```python
from build123d import *

# Parameters (mm, degrees)
RESSALTO_EXTRUS_O1_DEPTH = 3
ESBO_O2_R                = 2.5
RESSALTO_EXTRUS_O2_DEPTH = 18
ESBO_O3_R                = 0.85
CORTE_EXTRUS_O1_DEPTH    = 39.774991941
ESBO_O4_R                = 0.7
CORTE_EXTRUS_O2_DEPTH    = 38.235735524


with BuildPart() as part:
    # Esboço1 → Ressalto-extrusão1 (new body)
    with BuildSketch(Plane(origin=(0, 0, 0), x_dir=(0, 0, -1), z_dir=(1, 0, 0))):
        with BuildLine():
            Line((-30, 2.5), (30, 2.5))
            ThreePointArc((30, 2.5), (32.5, 0), (30, -2.5))
            Line((30, -2.5), (-30, -2.5))
            ThreePointArc((-30, -2.5), (-32.5, 0), (-30, 2.5))
        make_face()
    extrude(amount=RESSALTO_EXTRUS_O1_DEPTH)

    # Esboço2 → Ressalto-extrusão2 (add)
    with BuildSketch(Plane(origin=(3, 0, 0), x_dir=(0, 0, -1), z_dir=(1, 0, 0))):
        with Locations(Location((30, 0, 0), (0, 0, 90))):
            Circle(ESBO_O2_R)
    extrude(amount=RESSALTO_EXTRUS_O2_DEPTH)

    # Esboço3 → Corte-extrusão1 (cut, through all)
    with BuildSketch(Plane(origin=(21, 0, 0), x_dir=(0, 0, -1), z_dir=(1, 0, 0))):
        with Locations((30, 0)):
            Circle(ESBO_O3_R)
    extrude(amount=-CORTE_EXTRUS_O1_DEPTH, mode=Mode.SUBTRACT)

    # Esboço4 → Corte-extrusão2 (cut, through all)
    with BuildSketch(Plane(origin=(3, 0, 0), x_dir=(0, 0, -1), z_dir=(1, 0, 0))):
        with Locations((-30, 0)):
            Circle(ESBO_O4_R)
    extrude(amount=-CORTE_EXTRUS_O2_DEPTH, mode=Mode.SUBTRACT)


solid = part.part
```
Design review of the part built by this model. Coordinates are the model's own, in mm. A direction names the side the tool comes from. Give positions to 0.01 mm unless a question says otherwise; leave off trailing zeros. Order: outer loops, then holes, each group sorted by start corner. A loop starts at its lowest first (then second) coordinate and runs counter-clockwise, first axis right, second up. Notation, with made-up numbers: (-2.5, 59.5) -> (30.5, 59.5) arc R10 cw to (30.5, 77.5) -> close; hole circle Ø2 at (-27, -9). An arc over 180 degrees is marked (long way). Write each question's results on one line, items separated by ' | '. Start each with the question number.
Q1. For pin 1 (3 mm diameter, centred on x = 13, y = 0, fed in from +Z), flat-tipped, find the tip position at first contact; note if it passes through.
Q2. Machinability: for faces 4 (the cylindrical face through (10.65, 0.04, -29.15)), 5 (the cylindrical face through (10.35, -0.54, -32.44)), which of the approach directions +Z, -Z, +X, -X, +Y, -Y give a long, thin tool a straight path to every point of the face, cutting with its end or side? Answer none if there is none.
Q3. Mouldability with a two-part tool opening along Y and no side actions: class faces 1 (the cylindrical face through (1.521, 0.21, 29.332)), 2 (the flat face through (0, 0, 0)), 3 (the flat face through (1, -2.5, 0)) as +Y half, -Y half, draft (parallel to the pull), parting line (faces both ways), or undercut.
Q4. Add section B-B on x = 1.75. Give the boundary of the cut face in (y, z).
Q5. Add section C-C on x = 12.75. Give the boundary of the cut face in (y, z).
Q6. Wall thickness on L1, parallel to Y at x = 16.5, z = -30; L2, parallel to Z at x = 2.5, y = 0.35; L3, parallel to Y at x = 0.8, z = 30: over which ranges is each line inside the solid? List them lowest first. Write a range as from..to.
Q7. Add section D-D on z = -0.5. Give the boundary of the cut face in (x, y).
Q8. Add section A-A on y = 0. Give the boundary of the cut face in (x, z).
Found:
1) pin 1: stops at z = -27.5
2) face 4: +X, -X | face 5: +X
3) face 1: undercut | face 2: draft | face 3: -Y half
4) outline: (-2.5, -30) arc R2.5 ccw to (2.5, -30) -> (2.5, 30) arc R2.5 ccw to (-2.5, 30) -> close; hole circle Ø1.7 at (0, -30); hole circle Ø1.4 at (0, 30)
5) outline: circle Ø5 at (0, -30); hole circle Ø1.7 at (0, -30)
6) L1: y = -2.5..-0.85, 0.85..2.5 | L2: z = -32.48..-30.77, -29.23..29.39, 30.61..32.48 | L3: y = -2.5..-0.7, 0.7..2.5
7) outline: (0, -2.5) -> (3, -2.5) -> (3, 2.5) -> (0, 2.5) -> close
8) outline: (0, -32.5) -> (21, -32.5) -> (21, -30.85) -> (0, -30.85) -> close; (0, -29.15) -> (21, -29.15) -> (21, -27.5) -> (3, -27.5) -> (3, 29.3) -> (0, 29.3) -> close; (0, 30.7) -> (3, 30.7) -> (3, 32.5) -> (0, 32.5) -> close
